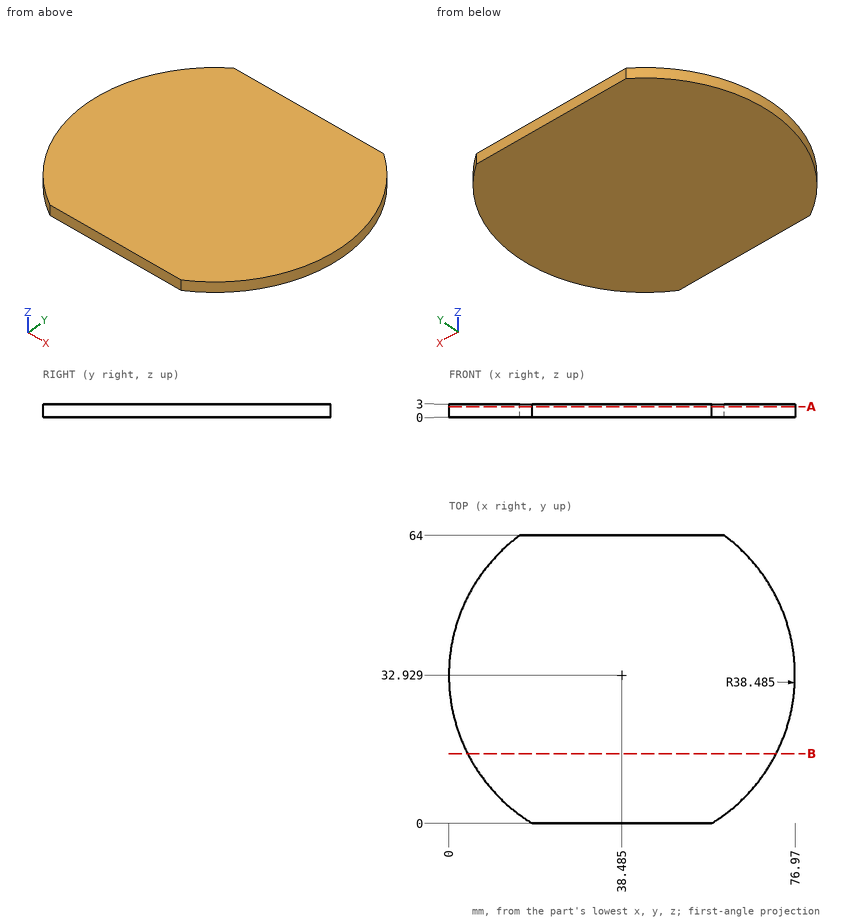
Study the drawing (mm; zero at the part's minimum x, y, z) and answer. Round coordinates to 2 decimals unless told otherwise and drop trailing zeros. Loops run counter-clockwise (first coordinate to the right, second up) from the corner with the lowest first, then second, coordinate; pieces in that order, holes last. Notation, with made-up numbers: M 72.5,30 L 77.5,30 A15 ccw 77.5,36 Z; hole C 11,-10.75 d8. An arc over 180 degrees is marked long. One line per question, with ' | ' between items.
Q1. Each of these flat-tipped pins is pushed along its axis until it touches: pin 1 Ø1.5 at (y, z) = (42.5, 2) entering from -X (1 decimal); pin 2 Ø1.5 at (x, y) = (46.5, 36) entering from -Z. Where does it stop, or does it pass through?
Conclusion:
pin 1: stops at x = 1 | pin 2: stops at z = 0
Q2. Find section A-A, the plane z = 2.4. Give the vertices of the cut face in (x, y) (1 decimal).
Conclusion:
outline: M 15.8,64 A38.5 ccw 18.6,0 L 58.4,0 A38.5 ccw 61.2,64 Z
Q3. Consider line 1 along Y through (x, z) = (61, 0.5); line 2 along X through (y, z) = (51.5, 2.35); line 3 along X through (y, z) = (26, 0.4). Determine where each line is inside the solid, lowest interval first. Write a range as from..to.
Conclusion:
line 1: y = 1.72..64 | line 2: x = 4.78..72.19 | line 3: x = 0.63..76.34
Q4. Find section B-B, the plane y = 15.5. Give the vertices of the cut face in (x, z), then the cut area to 3 significant figures.
Conclusion:
outline: M 4.17,0 L 72.8,0 L 72.8,3 L 4.17,3 Z | area: 206 mm2
